Work out the finished part from the listing and answer in its coordinate system (mm). Round coordinates to 2 decimals unless told otherwise and drop trailing zeros. Loops run counter-clockwise (first coordinate to the right, second up) from the corner with the lowest first, then second, coordinate; pieces in that order, holes last. Notation, with made-up numbers: M -6,0 L 29,0 A17 ccw 29,32 Z; hole C 55,38 d7. An arc over 180 degrees is marked long. One line per item, written item: value.
Autodesk Inventor part; units mm, degrees
ref_plane "YZ Plane" through (0, 0, 0) normal (1, 0, 0) x (0, 1, 0)
ref_plane "XZ Plane" through (0, 0, 0) normal (0, 1, 0) x (-1, 0, 0)
ref_plane "XY Plane" through (0, 0, 0) normal (0, 0, 1) x (1, 0, 0)
ref_plane "Work Plane2" through (0.4904, 0, 14) normal (0, 0, 1) x (1, 0, 0)
sketch "Sketch1" plane through (0.4904, 0, 14) normal (0, 0, 1) x (1, 0, 0)
  line L0 (-25, 245.7065) -> (25, 245.7065)
  line L1 (25, 245.7065) -> (25, 5.7065)
  line L2 (25, 5.7065) -> (-25, 5.7065)
  line L3 (-25, 5.7065) -> (-25, 245.7065)
  line L4 (-20, 245.7065) -> (20, 245.7065)
  line L5 (20, 5.7065) -> (-20, 5.7065)
  circle A0 centre (0, 30.7065) radius 3.5
  circle A1 centre (0, 30.7065) radius 25
  circle A2 centre (0, 245.7065) radius 20
  line L6 (-25, 30.7065) -> (-20, 245.7065)
  line L7 (20, 245.7065) -> (25, 30.7065)
  point P0 (-0.4904, 0)
  point P1 (-20, 245.7065)
  dimension "d6" = 240
  dimension "d7" = 0
  dimension "d9" = 50
  dimension "d10" = 25
  dimension "d11" = 25
  dimension "d12" = 25
  dimension "d13" = 0
extrude "Extrusion1" add sketch "Sketch1" along normal blind 3 contours A2 L0 | L0 A2 | A2 L7 A1 L6 | L6 A1 L7
sketch "Sketch2" plane through (0.4904, 0, 17) normal (0, 0, 1) x (1, 0, 0)
  arc A0 (20, 245.7065) -> (-20, 245.7065) centre (0, 245.7065) ccw
  circle A1 centre (0, 245.7065) radius 5
  point P0 (-0.4904, 0)
  dimension "d16" = 10
extrude "Extrusion2" cut sketch "Sketch2" against normal blind 3
sketch "Sketch3" plane through (0.4904, 0, 17) normal (0, 0, 1) x (1, 0, 0)
  circle A0 centre (-9.4508, 46.0264) radius 2.5
  circle A1 centre (8.7917, 14.9991) radius 2.5
  point P0 (-0.4904, 0)
extrude "Extrusion3" cut sketch "Sketch3" against normal blind 10
properties part number "Link2Base2"
1) Each of these flat-tipped pins is pushed along its axis until it touches: pin 1 (11 mm diameter, centred on x = 0.49, y = 30.71, fed in from +Z); pin 2 (1.5 mm diameter, centred on y = 65, z = 16.5, fed in from -X); pin 3 (1 mm diameter, centred on y = 155, z = 15, fed in from -X). Where does it stop, or does it pass through?
Check values:
pin 1: z = 17
pin 2: x = -23.73
pin 3: x = -21.63
2) Find section C-C (x = 9). Give the vertices of the cut face in (y, z).
Check values:
outline: M 7.2,14 L 12.52,14 L 12.52,17 L 7.2,17 Z; M 17.48,14 L 263.81,14 L 263.81,17 L 17.48,17 Z
3) The mould has two halves that part along X. Classify faces 1 (the face through (-0.594, 240.825, 15.521)), 2 (the face through (0.05, 265.7, 15.48)), 3 (the face through (0, 138, 14)): +X half, -X half, draft (parallel to the pull), parting line (faces both ways), or undercut.
Check values:
face 1: undercut
face 2: parting line
face 3: draft
4) Find section D-D (y = 179). Give the vertices of the cut face in (x, z), then the cut area to 3 significant figures.
Check values:
outline: M -21.06,14 L 22.04,14 L 22.04,17 L -21.06,17 Z
area: 129 mm2
5) Find section A-A (x = -9). Give the vertices of the cut face in (y, z), then the cut area to 3 significant figures.
Check values:
outline: M 7.58,14 L 43.53,14 L 43.53,17 L 7.58,17 Z; M 48.53,14 L 263.31,14 L 263.31,17 L 48.53,17 Z
area: 752 mm2
6) Find section B-B (z = 16.05). Give the vertices of the cut face in (x, y), then the cut area to 3 significant figures.
Check values:
outline: M -24.51,30.71 A25 ccw 25.49,30.71 L 20.49,245.71 A20 ccw -19.51,245.71 Z; hole C -8.96,46.03 d5; hole C 0.49,245.71 d10; hole C 0.49,30.71 d7; hole C 9.28,15 d5
area: 11,100 mm2
7) Find the intervals of material crossed by probe 1 along Y at (x, z) = (0.5, 16.75); probe 2 along Y at (x, z) = (-2, 14.2); probe 3 along Y at (x, z) = (9, 14.6), in increasing order. Write a range as from..to.
Check values:
probe 1: 5.71..27.21, 34.21..240.71, 250.71..265.71
probe 2: 5.83..28.25, 33.17..241.37, 250.04..265.55
probe 3: 7.2..12.52, 17.48..263.81
